Could you check a few things on this model? Use its own coordinates, in mm. A direction names the side the tool comes from. Give positions to 0.01 mm unless a question says otherwise; leave off trailing zeros. Loops run counter-clockwise (first coordinate to the right, second up) from the corner with the lowest first, then second, coordinate; pieces in that order, holes last. Notation, with made-up numbers: M 41,45 L 98,45 A12 ccw 98,54 Z; hole C 69.5,-11 d8. An arc over 180 degrees is marked long. Return JSON: item names as keys, results as strings. Group by question number.
1. For faces 1 (the flat face through (7, -39, -11.702)), 2 (the flat face through (10, -35, 0)), which set-ups out of +Z, -Z, +X, -X, +Y, -Y let a thin tool reach every point of the face, with its end or its side?
2. Please list where these lines run through material, in increasing order: line 1 (Y direction, x = 3.5, z = 0) (3 decimals); line 2 (X direction, y = -28.5, z = 7.75); line 3 (Y direction, x = 15.25, z = 4.75).
3. If we mould it in two halves opening along Z, with no side actions, what happens to faces 3 (the flat face through (7, -39, 12.298)), 4 (the cylindrical face through (4.93, -8.53, 1.89)), 5 (the flat face through (12, -88.573, 0))? For each: +Z half, -Z half, draft (parallel to the pull), parting line (faces both ways), or undercut.
4. If we section it at D-D (y = -21.5): Write out the boundary of the cut face in (x, z).
5. If we section it at A-A (z = 0): Write out the boundary of the cut face in (x, y) (3 decimals).
6. For pin 1 (6 mm diameter, centred on x = 18, z = 9.5, fed in from +Y); pin 2 (5 mm diameter, centred on y = -37, z = 5.5, fed in from -X); pin 3 (7 mm diameter, centred on y = -56, z = 4.5, fed in from +X), each with a flat end and sliding along its axis, tell me the tip position at first contact or that it passes through.
7. If we section it at C-C (z = 11.25): Write out the boundary of the cut face in (x, y).
8. If we section it at B-B (x = 2.25): Write out the boundary of the cut face in (y, z) (3 decimals), plus the area to 3 significant figures.
```python
from build123d import *

# Parameters (mm, degrees)
SKETCH1_W           = 24
SKETCH1_H           = 100
SKETCH1_R           = 8.735
BOSS_EXTRUDE1_DEPTH = 10
SKETCH2_W           = 24
SKETCH2_H           = 6.573473922
BOSS_EXTRUDE2_DEPTH = 15


with BuildPart() as part:
    # Sketch1 → Boss-Extrude1 (new body)
    with BuildSketch(Plane(origin=(0, 0, 0), x_dir=(0, 0, -1), z_dir=(1, 0, 0))):
        with Locations((-0.298142376, -38.573473922)):
            Rectangle(SKETCH1_W, SKETCH1_H)
        Circle(SKETCH1_R, mode=Mode.SUBTRACT)
    extrude(amount=BOSS_EXTRUDE1_DEPTH)

    # Sketch2 → Boss-Extrude2 (add)
    with BuildSketch(Plane(origin=(10, 0, 0), x_dir=(0, 0, -1), z_dir=(1, 0, 0))):
        with Locations((-0.298142376, -85.286736961)):
            Rectangle(SKETCH2_W, SKETCH2_H)
    extrude(amount=BOSS_EXTRUDE2_DEPTH)


solid = part.part
```
Answer:
{
 "1": {"face 1": "-Z, +X, -X, +Y, -Y", "face 2": "+Z, -Z, +X, +Y"},
 "2": {"line 1": "y = -88.573 to -8.735, 8.735 to 11.427", "line 2": "x = 0 to 10", "line 3": "y = -88.57 to -82"},
 "3": {"face 3": "+Z half", "face 4": "undercut", "face 5": "draft"},
 "4": {"outline": "M 0,-11.7 L 10,-11.7 L 10,12.3 L 0,12.3 Z"},
 "5": {"outline": "M 0,-88.573 L 25,-88.573 L 25,-82 L 10,-82 L 10,-8.735 L 0,-8.735 Z; M 0,8.735 L 10,8.735 L 10,11.427 L 0,11.427 Z"},
 "6": {"pin 1": "stops at y = -82", "pin 2": "stops at x = 0", "pin 3": "stops at x = 10"},
 "7": {"outline": "M 0,-88.57 L 25,-88.57 L 25,-82 L 10,-82 L 10,11.43 L 0,11.43 Z"},
 "8": {"outline": "M -88.573,-11.702 L 11.427,-11.702 L 11.427,12.298 L -88.573,12.298 Z; hole C 0,0 d17.47", "area": "2,160 mm²"}
}
